Can you work these out from the model? Positions are in its coordinate system, mm. A direction names the side the tool comes from. Coordinates: 2 decimals unless noted, no trailing zeros. Loops run counter-clockwise (first coordinate to the right, second up) from the corner with the lowest first, then second, coordinate; pieces in that order, holes last.
```python
from build123d import *

# Parameters (mm, degrees)
F0_W     = 25.4
F0_H     = 4.7498
F0_H_2   = 4.7752
F0_H_3   = 19.05
F1_DEPTH = 25.4
F2_DEPTH = 63.5
F3_DEPTH = 12.7


with BuildPart() as f1:
    # F0 (on Front) → F1 (new body, symmetric)
    with BuildSketch(Plane.XZ):
        with Locations((73.025, 64.3001)):
            Rectangle(F0_W, F0_H)
        with Locations((73.025, 40.4876)):
            Rectangle(F0_W, F0_H_2)
        with BuildLine():
            Line((22.225, 9.525), (41.275, 9.525))
            Line((41.275, 9.525), (41.275, 27.0002))
            ThreePointArc((41.275, 27.0002), (45.9246798487, 38.2255201513), (57.15, 42.8752))
            Line((57.15, 42.8752), (60.325, 42.8752))
            Line((60.325, 42.8752), (60.325, 61.9252))
            Line((60.325, 61.9252), (57.15, 61.9252))
            add(Edge.make_bspline(
                [(55.0049951234, 61.8592673868), (55.7203693302, 61.8825211743), (56.4354212261, 61.9044283334), (57.15, 61.9252)],
                knots=[109.5299309045, 109.5299309045, 109.5299309045, 109.5299309045, 111.5045361635, 111.5045361635, 111.5045361635, 111.5045361635], degree=3))
            ThreePointArc((55.0049951234, 61.8592673868), (31.7072218467, 50.9255143102), (22.225, 27.0002))
            Line((22.225, 27.0002), (22.225, 9.525))
        make_face()
        with Locations((73.025, 52.4002)):
            Rectangle(F0_W, F0_H_3)
        Polygon((85.725, 61.9252), (85.725, 42.8752), (85.725, 38.1), (111.125, 38.1), (111.125, 66.675), (85.725, 66.675), align=None)
        with BuildLine():
            ThreePointArc((57.15, 61.9252), (56.0769910263, 61.9087129552), (55.0049951234, 61.8592673868))
            add(Edge.make_bspline(
                [(55.0049951234, 61.8592673868), (55.7203693302, 61.8825211743), (56.4354212261, 61.9044283334), (57.15, 61.9252)],
                knots=[109.5299309045, 109.5299309045, 109.5299309045, 109.5299309045, 111.5045361635, 111.5045361635, 111.5045361635, 111.5045361635], degree=3))
        make_face()
        Polygon((41.275, -9.525), (41.275, 9.525), (22.225, 9.525), (-41.275, 9.525), (-41.275, -9.525), align=None)
    extrude(amount=F1_DEPTH, both=True)

    # F2 (add, symmetric): a face of the model
    f2_faces = [f1.faces().sort_by_distance(p)[0] for p in [
        (40.4852696712, -25.4, 28.4092448442),
    ]]
    extrude(f2_faces, amount=F2_DEPTH, both=True)

    # F3 (add, symmetric): a face of the model
    f3_faces = [f1.faces().sort_by_distance(p)[0] for p in [
        (40.4852696712, -88.9, 28.4092448442),
    ]]
    extrude(f3_faces, amount=F3_DEPTH, both=True)


solid = f1.part
```
(1) I want a section at C-C on x = 87.5. Write out the boundary of the cut face in (y, z) (3 decimals).
Check values:
outline: (-101.6, 38.1) - (38.1, 38.1) - (38.1, 66.675) - (-101.6, 66.675) - close
(2) I want a section at D-D on z = 12.5. Write out the boundary of the cut face in (x, y) (3 decimals).
Check values:
outline: (22.225, -101.6) - (41.275, -101.6) - (41.275, 38.1) - (22.225, 38.1) - close
(3) If I drill on probe 1 along X at (y, z) = (-12, 10) (3 decimals); probe 2 along Z at (x, y) = (19, -44) (3 decimals); probe 3 along X at (y, z) = (-77.5, 39.5) (3 decimals), over which ranges is the centre line in solid material (lowest first)?
Check values:
probe 1: x = 22.225 to 41.275
probe 2: z = -9.525 to 9.525
probe 3: x = 24.538 to 47.364, 60.325 to 111.125
(4) I want a section at A-A on y = -87.5. Write out the boundary of the cut face in (x, z) (3 decimals).
Check values:
outline: (-41.275, -9.525) - (41.275, -9.525) - (41.275, 27) arc R15.875 cw to (57.15, 42.875) - (60.325, 42.875) - (60.325, 38.1) - (111.125, 38.1) - (111.125, 66.675) - (60.325, 66.675) - (60.325, 61.925) - (57.15, 61.925) arc R34.925 ccw to (22.225, 27) - (22.225, 9.525) - (-41.275, 9.525) - close
(5) Which directions (+Z, -Z, +X, -X, +Y, -Y) give clear straight access to the entire face, cutting with the end or side of a thin tool? Please do faces 4 (the flat face through (-1, -33, -9.525)), 5 (the flat face through (60.325, -33, 40)), 6 (the flat face through (41.275, -33, 8)), 7 (the flat face through (111.125, -33, 52)), 8 (the flat face through (-9, -33, 9.525)).
Check values:
face 4: -Z, +X, -X, +Y, -Y
face 5: -Z, +Y, -Y
face 6: -Z, +X, +Y, -Y
face 7: +Z, -Z, +X, +Y, -Y
face 8: +Z, -X, +Y, -Y
(6) If we mould it in two halves opening along X, with no side actions, what happens to faces 1 (the flat face through (85, -33, 38.1)), 2 (the flat face through (60.325, -33, 64)), 3 (the cylindrical face through (45.8, -32.7, 38.1))? For each: released by +X, released by -X, zero draft, split by the parting line, or undercut.
Check values:
face 1: zero draft
face 2: released by -X
face 3: undercut
(7) I'm going to push flat-ended pins straight in: pin 1 (5.5 mm diameter, centred on y = -54, z = 41, fed in from -X); pin 2 (5 mm diameter, centred on y = -13, z = 21.5, fed in from -X) (3 decimals); pin 3 (1.6 mm diameter, centred on x = 59, y = -65.5, fed in from +Z). Where does each tip first touch, or does it pass through?
Check values:
pin 1: stops at x = 24.09
pin 2: stops at x = 22.225
pin 3: stops at z = 61.93
(8) I want a section at B-B on z = 41. Write out the boundary of the cut face in (x, y) (3 decimals).
Check values:
outline: (25.154, -101.6) - (49.665, -101.6) - (49.665, 38.1) - (25.154, 38.1) - close; (60.325, -101.6) - (111.125, -101.6) - (111.125, 38.1) - (60.325, 38.1) - close
